Source: CAD feature listing. Evaluate the final solid. Frame: model axes, mm. A direction names the side the tool comes from. Give positions to 0.01 mm unless a question says otherwise; leave off trailing zeros. Order: outer loops, then holes, each group sorted by start corner. A loop starts at its lowest first (then second) coordinate and runs counter-clockwise, first axis right, second up.
Autodesk Inventor part; units mm, degrees
ref_plane "YZ Plane" through (0, 0, 0) normal (1, 0, 0) x (0, 1, 0)
ref_plane "XZ Plane" through (0, 0, 0) normal (0, 1, 0) x (-1, 0, 0)
ref_plane "XY Plane" through (0, 0, 0) normal (0, 0, 1) x (1, 0, 0)
sketch "Sketch1" plane through (0, 0, 0) normal (0, 0, 1) x (1, 0, 0)
  circle A0 centre (0, 0) radius 9.9949
  line L0 (0, 0) -> (-4.7625, 0)
  line L1 (-4.7625, 2.7354) -> (-0.0123, 5.4921)
  line L2 (-0.0123, 5.4921) -> (4.7502, 2.7568)
  line L3 (4.7502, 2.7568) -> (4.7625, -2.7354)
  line L4 (4.7625, -2.7354) -> (0.0123, -5.4921)
  line L5 (0.0123, -5.4921) -> (-4.7502, -2.7568)
  line L6 (-4.7502, -2.7568) -> (-4.7625, 2.7354)
  dimension "d1" = 19.9898
  dimension "d4" = 4.7625
extrude "Extrusion2" add sketch "Sketch1" along normal blind 1.5875
properties part number "Spacer 1 16 in"
1) Section query A-A on z = 1.35. Output: boundary loops of the cut face in (x, y).
Checks:
outline: circle Ø19.99 at (0, 0); hole (-4.76, 2.74) - (-4.75, -2.76) - (0.01, -5.49) - (4.76, -2.74) - (4.75, 2.76) - (-0.01, 5.49) - close
2) First-contact query: pin 1 Ø5 at (x, y) = (6, 2) entering from -Z. Flat tip, straight axial feed; report the tip coordinate or a pass-through.
Checks:
pin 1: stops at z = 0
3) Section query B-B on y = -4.25. Output: boundary loops of the cut face in (x, z).
Checks:
outline: (-9.05, 0) - (-2.15, 0) - (-2.15, 1.59) - (-9.05, 1.59) - close; (2.15, 0) - (9.05, 0) - (9.05, 1.59) - (2.15, 1.59) - close
4) Reachability of faces 1 (the face through (-2.34, -4.14, 0.78)), 2 (the face through (-2.4, -4.3, 0)) from +Z, -Z, +X, -X, +Y, -Y: full face, straight path, thin tool, end or side. Return the list, or none.
Checks:
face 1: +Z, -Z
face 2: -Z, +X, -X, +Y, -Y
5) Section query C-C on x = 2.75. Output: boundary loops of the cut face in (y, z), and give its area (3 significant figures).
Checks:
outline: (-9.61, 0) - (-3.9, 0) - (-3.9, 1.59) - (-9.61, 1.59) - close; (3.91, 0) - (9.61, 0) - (9.61, 1.59) - (3.91, 1.59) - close
area: 18.1 mm2
6) Pull-direction query (X, two-part tool) for faces 3 (the face through (-2.421, 4.094, 0.783)), 4 (the face through (9.533, -3.002, 0.783)), 5 (the face through (-2.4, -4.3, 1.588)), 6 (the face through (2.421, -4.094, 0.783)); classes: +X half, -X half, draft (parallel to the pull), parting line (faces both ways), or undercut.
Checks:
face 3: undercut
face 4: parting line
face 5: draft
face 6: undercut
7) Ray query, L1, parallel to Y at x = 1.25, z = 0.65; L2, parallel to Y at x = -0.75, z = 1.25; L3, parallel to X at y = -2.5, z = 1.05. Return the intervals inside material, ascending.
Checks:
L1: y = -9.92 to -4.77, 4.77 to 9.92
L2: y = -9.97 to -5.05, 5.06 to 9.97
L3: x = -9.68 to -4.75, 4.76 to 9.68
8) Section query D-D on x = 8.25. Output: boundary loops of the cut face in (y, z).
Checks:
outline: (-5.64, 0) - (5.64, 0) - (5.64, 1.59) - (-5.64, 1.59) - close
